Geometry check sheet. Reference: the model listing, model coordinates, mm. A direction names the side the tool comes from. Coordinates: 2 decimals unless noted, no trailing zeros. Write each loop counter-clockwise with the first axis right and the second up, starting at its lowest first coordinate (ties: lowest second). Pieces come first, ordered by that corner, then holes. Notation, with made-up numbers: (-1.75, 49.25) -> (9.25, 49.25) arc R25 ccw to (9.25, 76.25) -> close; hole circle Ø4 at (65, 67). An arc over 180 degrees is marked (long way). Answer in a Markdown table with one row per item. Add a question column.
Q1. Section check D-D, the plane y = -13. Count the separate pieces of the cut face and the enclosed holes in it, and give its area (3 significant figures).
Q2. Section check C-C, the plane z = 6.5. Record the boundary of the cut face in (x, y), and give its area (3 significant figures).
Q3. Section check A-A, the plane x = -20. Record the boundary of the cut face in (y, z).
Q4. Tool access check on faces 1 (the face through (-92.5, -15, 0)), 2 (the face through (-1, -82.46, 0)). Record the directions out of +Z, -Z, +X, -X, +Y, -Y that give a thin tool (end or side, any length) a straight path to the whole face; none if there is none.
Q5. Thickness scan on line 1 (Z direction, x = 8, y = -44); line 2 (Z direction, x = -51.5, y = -38); line 3 (X direction, y = -42, z = 15.5). Record the ranges inside material, lowest first.
Q6. Gauge pin test, flat ends, axial feed: P1, Ø1, axis at y = -59, z = -36, coming from the +X side; P2, Ø5, axis at y = -45.5, z = 13, coming from the -X side; P3, Ø1.6, axis at y = -59, z = 36, coming from the +X side. Record the tip position at first contact, or that the pin passes through.
Q7. Release check for a two-part mould opening along X. For faces 3 (the face through (-89.96, -15, 0)), 4 (the face through (-88.06, -18.99, 35.46)), 5 (the face through (89.73, -37.38, 0.56)), 6 (the face through (31, -63, 37)) record: pulls with the +X half, pulls with the -X half, needs draft (parallel to the pull), parting line crosses it, or undercut.
```python
from build123d import *

# Parameters (mm, degrees)
F0_W        = 185
F0_H        = 80
F1_DEPTH    = 40
F2_W        = 125
F2_H        = 70
F3_DEPTH    = 45
F4_R        = 9.1981536726
F5_T        = 2.54
F5_T3_DEPTH = 130.08
F5_T5_DEPTH = 75.08
F7_DEPTH    = 112.6
F8_W        = 49.0510910749
F8_H        = 28.2043814659
F8_W_2      = 47.2116749734
F9_DEPTH    = 2
F10_W       = 52.2382371128
F10_H       = 31.3754677773
F10_W_2     = 46.3282726705
F10_H_2     = 29.9284607172
F11_DEPTH   = 2
F12_W       = 31.3480645418
F12_H       = 61.4709071815
F13_DEPTH   = 2
F14_W       = 33.0155193806
F14_H       = 60.6432519853
F15_DEPTH   = 2


# Not quite as in the source:
# - a shell that OpenCascade refuses in one call is made with other operations: the cavity is built on its own and cut out


with BuildPart() as f1:
    # F0 (on Front) → F1 (new body)
    with BuildSketch(Plane.XZ):
        Rectangle(F0_W, F0_H)
    extrude(amount=F1_DEPTH)

    # F2 (on face) → F3 (join)
    with BuildSketch(Plane.XZ.offset(40)):
        Rectangle(F2_W, F2_H)
    extrude(amount=F3_DEPTH)

    # F4
    f4_edges = [f1.edges().sort_by_distance(p)[0] for p in [
        (-92.5, -40, 0),
        (92.5, -40, 0),
        (92.5, -20, 40),
        (92.5, -20, -40),
        (-92.5, -20, -40),
        (-92.5, -20, 40),
    ]]
    fillet(f4_edges, radius=F4_R)

    # F5: shell of thickness 2.54, made by hand


with BuildPart() as f5_core1:
    # F5_t2: copy of F1
    add(f1.part)

    # the walls: a layer under each face that stays
    f5_faces = [f5_core1.faces().sort_by_distance(p)[0] for p in [
        (0, -20, 40),
        (89.8059231637, -20, 37.3059231637),
        (-89.8059231637, -20, 37.3059231637),
        (-71.4015825663, -40, -34.2857142857),
        (92.5, -15.4009231637, 0),
        (-92.5, -15.4009231637, 0),
        (89.8059231637, -20, -37.3059231637),
        (-89.8059231637, -20, -37.3059231637),
        (0, -20, -40),
        (89.8059231637, -37.3059231637, 0),
        (-89.8059231637, -37.3059231637, 0),
        (0, -62.5, 35),
        (-62.5, -62.5, 0),
        (0, -62.5, -35),
        (62.5, -62.5, 0),
        (0, -85, 0),
    ]]
    thicken(f5_faces, amount=-F5_T, mode=Mode.SUBTRACT)

    # F5_s4 → F5_t3 (cut)
    with BuildSketch(Plane.YZ.offset(-65.04)):
        Polygon((-40.0254, 35.0254), (-37.46, 35), (-37.46, 32.46), (-40, 32.46), align=None)
        Polygon((-40.0254, -35.0254), (-37.46, -35), (-37.46, -32.46), (-40, -32.46), align=None)
    extrude(amount=F5_T3_DEPTH, mode=Mode.SUBTRACT)

    # F5_s6 → F5_t5 (cut)
    with BuildSketch(Plane.XY.offset(-37.54)):
        Polygon((-62.5254, -40.0254), (-62.5, -37.46), (-59.96, -37.46), (-59.96, -40), align=None)
        Polygon((62.5254, -40.0254), (62.5, -37.46), (59.96, -37.46), (59.96, -40), align=None)
    extrude(amount=F5_T5_DEPTH, mode=Mode.SUBTRACT)


with BuildPart() as f1_1:
    add(f1.part)

    # what is left inside the walls is the cavity
    f5_cavity = [f5_core1.part.solids().sort_by_distance(p)[0] for p in [
        (0, -0.0254, -12.486667),
    ]]
    add(f5_cavity, mode=Mode.SUBTRACT)

    # F6 (on face) → F7 (cut)
    with BuildSketch(Plane.XY.offset(40)):
        with BuildLine():
            ThreePointArc((-66.3535060933, 0), (-47.3649650812, -18.9885410121), (-28.3764240691, 0))
            Line((-28.3764240691, 0), (-66.3535060933, 0))
        make_face()
        with BuildLine():
            Line((64.9945122235, 0), (29.1222798593, 0))
            ThreePointArc((29.1222798593, 0), (47.0583960414, -17.9361161821), (64.9945122235, 0))
        make_face()
    extrude(amount=-F7_DEPTH, mode=Mode.SUBTRACT)

    # F8 (on face) → F9 (join)
    with BuildSketch(Plane(origin=(0, 0, -35), x_dir=(1, 0, 0), z_dir=(0, 0, -1))):
        with Locations((-31.4233601093, 61.8686154485)):
            Rectangle(F8_W, F8_H)
        with Locations((32.0364944637, 61.8686154485)):
            Rectangle(F8_W_2, F8_H)
    extrude(amount=F9_DEPTH)

    # F10 (on face) → F11 (join)
    with BuildSketch(Plane.XY.offset(35)):
        with Locations((30.9228170663, -63.50582093)):
            Rectangle(F10_W, F10_H)
        with Locations((-33.6980968714, -63.50582093)):
            Rectangle(F10_W_2, F10_H_2)
    extrude(amount=F11_DEPTH)

    # F12 (on face) → F13 (join)
    with BuildSketch(Plane(origin=(-62.5, 0, 0), x_dir=(0, -1, 0), z_dir=(-1, 0, 0))):
        with Locations((62.5, 0)):
            Rectangle(F12_W, F12_H)
    extrude(amount=F13_DEPTH)

    # F14 (on face) → F15 (join)
    with BuildSketch(Plane.YZ.offset(62.5)):
        with Locations((-62.5, 0)):
            Rectangle(F14_W, F14_H)
    extrude(amount=F15_DEPTH)


solid = f1_1.part
```
Calculated:
| question | item | result |
|---|---|---|
| 1 | separate pieces | 4 |
| 1 | enclosed holes | 0 |
| 1 | area | 1,020 mm² |
| 2 | outline | (-92.5, -30.8) arc R9.2 ccw to (-83.3, -40) -> (-62.5, -40) -> (-62.5, -46.83) -> (-64.5, -46.83) -> (-64.5, -78.17) -> (-62.5, -78.17) -> (-62.5, -85) -> (62.5, -85) -> (62.5, -79.01) -> (64.5, -79.01) -> (64.5, -45.99) -> (62.5, -45.99) -> (62.5, -40) -> (83.3, -40) arc R9.2 ccw to (92.5, -30.8) -> (92.5, 0) -> (89.96, 0) -> (89.96, -30.8) arc R6.66 cw to (83.3, -37.46) -> (59.96, -37.46) -> (59.96, -82.46) -> (-59.96, -82.46) -> (-59.96, -37.46) -> (-83.3, -37.46) arc R6.66 cw to (-89.96, -30.8) -> (-89.96, 0) -> (-92.5, 0) -> close |
| 2 | area | 1,000 mm² |
| 3 | outline | (-85, -35) -> (-75.97, -35) -> (-75.97, -37) -> (-47.77, -37) -> (-47.77, -35) -> (-40, -35) -> (-40, -40) -> (0, -40) -> (0, -37.46) -> (-37.46, -37.46) -> (-37.46, -32.46) -> (-82.46, -32.46) -> (-82.46, 32.46) -> (-37.46, 32.46) -> (-37.46, 37.46) -> (0, 37.46) -> (0, 40) -> (-40, 40) -> (-40, 35) -> (-48.54, 35) -> (-48.54, 37) -> (-78.47, 37) -> (-78.47, 35) -> (-85, 35) -> close |
| 4 | face 1 | +Z, -Z, -X, +Y, -Y |
| 4 | face 2 | +Y |
| 5 | line 1 | z = -35 to -32.46, 32.46 to 35 |
| 5 | line 2 | z = -40 to -32.46, 32.46 to 40 |
| 5 | line 3 | x = -62.5 to -59.96, 59.96 to 62.5 |
| 6 | P1 | stops at x = 55.64 |
| 6 | P2 | stops at x = -64.5 |
| 6 | P3 | stops at x = 57.04 |
| 7 | face 3 | undercut |
| 7 | face 4 | undercut |
| 7 | face 5 | pulls with the +X half |
| 7 | face 6 | needs draft |
